```python
from build123d import *

# Parameters (mm, degrees)
SKETCH1_R           = 22.4995417
SKETCH1_R_2         = 17.4995417
BOSS_EXTRUDE1_DEPTH = 6
CUT_EXTRUDE1_START  = -4
SKETCH2_R           = 19.4995417
SKETCH2_R_2         = 17.4995417
CUT_EXTRUDE1_DEPTH  = 4
BOSS_EXTRUDE2_DEPTH = 6
BOSS_EXTRUDE3_START = 24
BOSS_EXTRUDE3_DEPTH = 24
BOSS_EXTRUDE4_START = 5
SKETCH6_R           = 22.4995417
SKETCH6_R_2         = 8.79453705
BOSS_EXTRUDE4_DEPTH = 5
CUT_EXTRUDE2_DEPTH  = 50
SKETCH8_W           = 26.34206851
SKETCH8_H           = 62.78523096
CUT_EXTRUDE3_DEPTH  = 44.051814752
SKETCH9_R           = 2.165
CUT_EXTRUDE4_DEPTH  = 33.379912807


with BuildPart() as part:
    # Sketch1 → Boss-Extrude1 (new body)
    with BuildSketch(Plane.XY):
        Circle(SKETCH1_R)
        Circle(SKETCH1_R_2, mode=Mode.SUBTRACT)
    extrude(amount=BOSS_EXTRUDE1_DEPTH)

    # Sketch2 → Cut-Extrude1 (cut)
    with BuildSketch(Plane.XY.offset(6).offset(CUT_EXTRUDE1_START)):
        Circle(SKETCH2_R)
        Circle(SKETCH2_R_2, mode=Mode.SUBTRACT)
    extrude(amount=CUT_EXTRUDE1_DEPTH, mode=Mode.SUBTRACT)

    # Sketch3 → Boss-Extrude2 (add, through all)
    with BuildSketch(Plane(origin=(0, 0, 0), x_dir=(-1, 0, 0), z_dir=(0, 0, -1))):
        with BuildLine():
            Line((-7.783576547, 21.11031295), (-21.864631522, 21.11031295))
            Line((-21.864631522, 21.11031295), (-21.864631522, 5.307284156))
            ThreePointArc((-21.864631522, 5.307284156), (-16.798452018, 14.96801211), (-7.783576547, 21.11031295))
        make_face()
        with BuildLine():
            Line((21.864631522, -21.11031295), (7.783576547, -21.11031295))
            ThreePointArc((7.783576547, -21.11031295), (16.798452018, -14.96801211), (21.864631522, -5.307284156))
            Line((21.864631522, -5.307284156), (21.864631522, -21.11031295))
        make_face()
        with BuildLine():
            Line((21.864631522, 21.11031295), (7.783576547, 21.11031295))
            ThreePointArc((7.783576547, 21.11031295), (16.798452018, 14.96801211), (21.864631522, 5.307284156))
            Line((21.864631522, 5.307284156), (21.864631522, 21.11031295))
        make_face()
        with BuildLine():
            Line((-21.864631522, -21.11031295), (-21.864631522, -5.307284156))
            ThreePointArc((-21.864631522, -5.307284156), (-16.798452018, -14.96801211), (-7.783576547, -21.11031295))
            Line((-7.783576547, -21.11031295), (-21.864631522, -21.11031295))
        make_face()
    extrude(amount=-BOSS_EXTRUDE2_DEPTH)

    # Sketch5 → Boss-Extrude3 (add)
    with BuildSketch(Plane(origin=(0, 0, 0), x_dir=(-1, 0, 0), z_dir=(0, 0, -1)).offset(BOSS_EXTRUDE3_START)):
        with BuildLine():
            Line((-14.441527519, 9.883129191), (-18.5677863, 12.706954341))
            ThreePointArc((-18.5677863, 12.706954341), (-22.4995417, 0), (-18.5677863, -12.706954341))
            Line((-18.5677863, -12.706954341), (-14.441527519, -9.883129191))
            ThreePointArc((-14.441527519, -9.883129191), (-17.4995417, 0), (-14.441527519, 9.883129191))
        make_face()
    extrude(amount=-BOSS_EXTRUDE3_DEPTH)

    # Sketch6 → Boss-Extrude4 (add)
    with BuildSketch(Plane(origin=(0, 0, -24), x_dir=(-1, 0, 0), z_dir=(0, 0, -1)).offset(BOSS_EXTRUDE4_START)):
        Circle(SKETCH6_R)
        Circle(SKETCH6_R_2, mode=Mode.SUBTRACT)
    extrude(amount=-BOSS_EXTRUDE4_DEPTH)

    # Sketch7 → Cut-Extrude2 (cut, symmetric)
    with BuildSketch(Plane(origin=(0, 0, 0), x_dir=(-1, 0, 0), z_dir=(0, 0, -1))):
        Polygon((0, 20.425006128), (0, -31.813494394), (-34.413040629, -24.963896379), (-30.369302041, 32.308646058), (-0.660202218, 29.585311907), (0, 25.789149152), align=None)
    extrude(amount=CUT_EXTRUDE2_DEPTH, both=True, mode=Mode.SUBTRACT)


with BuildPart() as cut_extrude2_piece_1:
    # of the separate pieces the step leaves, piece 1, a body of its own (cut_extrude2_pieces)
    add(part.part.solids().sort_by_distance((0, -22.4995417, -24))[0])

    # Sketch8 → Cut-Extrude3 (cut, through all)
    with BuildSketch(Plane(origin=(0, 0, 0), x_dir=(0, 0, -1), z_dir=(1, 0, 0))):
        with Locations((23.482670262, -0.940788161)):
            Rectangle(SKETCH8_W, SKETCH8_H)
    extrude(amount=-CUT_EXTRUDE3_DEPTH, mode=Mode.SUBTRACT)


with BuildPart() as cut_extrude2_piece_2:
    # of the separate pieces the step leaves, piece 2, a body of its own (cut_extrude2_pieces)
    add(part.part.solids().sort_by_distance((0, 17.4995417, 0))[0])

    # Sketch9 → Cut-Extrude4 (cut, through all)
    with BuildSketch(Plane(origin=(0, 0, 0), x_dir=(-1, 0, 0), z_dir=(0, 0, -1))):
        with Locations((16.571715691, 16)):
            Circle(SKETCH9_R)
        with Locations((16.571715691, -16)):
            Circle(SKETCH9_R)
        with Locations((-16.571715691, -16)):
            Circle(SKETCH9_R)
        with Locations((-16.571715691, 16)):
            Circle(SKETCH9_R)
    extrude(amount=-CUT_EXTRUDE4_DEPTH, mode=Mode.SUBTRACT)


solid = cut_extrude2_piece_2.part
```
Check sheet for the modelled part. Datum: model origin and axes. Units: mm. A direction names the side the tool comes from. Round coordinates to 2 decimals unless told otherwise and drop trailing zeros. Order: outer loops, then holes, each group sorted by start corner. A loop starts at its lowest first (then second) coordinate and runs counter-clockwise, first axis right, second up. Notation, with made-up numbers: M 22,58.5 L 61,58.5 A14 ccw 61,66.5 Z; hole C -39.75,47 d7. An arc over 180 degrees is marked long. Answer in a Markdown table with one row per item.
(1) Gauge pin test, flat ends, axial feed: pin 1 (2 mm diameter, centred on x = -11.5, z = 2, fed in from -Y); pin 2 (1.8 mm diameter, centred on y = -9.5, z = 3, fed in from -X); pin 3 (2 mm diameter, centred on y = 3, z = 1.5, fed in from -X); pin 4 (3.5 mm diameter, centred on x = -16.57, y = 16, fed in from -Z). Record the tip position at first contact, or that the pin passes through.
Findings:
| item | result |
|---|---|
| pin 1 | stops at y = -21.11 |
| pin 2 | stops at x = -21.86 |
| pin 3 | stops at x = -22.41 |
| pin 4 | passes through |
(2) Section check D-D on y = 0. Record the boundary of the cut face in (x, z), plus the area to 3 significant figures.
Findings:
| item | result |
|---|---|
| outline | M -22.5,0 L -17.5,0 L -17.5,2 L -19.5,2 L -19.5,6 L -22.5,6 Z |
| area | 22.0 mm^2 |
(3) Material ranges on line 1 along Y through (x, z) = (-15, 3.75); line 2 along Y through (x, z) = (-16, 2.2); line 3 along Y through (x, z) = (-20.75, 4.25), recorded low to high. Write a range as from..to.
Findings:
| item | result |
|---|---|
| line 1 | y = -21.11..-17.49, -14.51..-12.46, 12.46..14.51, 17.49..21.11 |
| line 2 | y = -21.11..-18.09, -13.91..-11.15, 11.15..13.91, 18.09..21.11 |
| line 3 | y = -21.11..21.11 |
(4) Draft check along Y on faces 1 (the cylindrical face through (-17.495, 0.385, 0.986)), 2 (the flat face through (-15, 21.11, 3)), 3 (the flat face through (-15, -21.11, 3)), 4 (the flat face through (-19, 0, 0)). Enter one of: +Y half, -Y half, draft (parallel to the pull), parting line (faces both ways), or undercut.
Findings:
| item | result |
|---|---|
| face 1 | undercut |
| face 2 | +Y half |
| face 3 | -Y half |
| face 4 | draft |
(5) Set-up check for faces 5 (the flat face through (-21.865, 13, 3)), 6 (the flat face through (-21.865, -13, 3)), 7 (the cylindrical face through (-22.5, 0.1, 3)), 8 (the cylindrical face through (-19.495, 0.429, 3.972)): record each of +Z, -Z, +X, -X, +Y, -Y from which the full face is reachable in a straight line by a thin tool's end or side.
Findings:
| item | result |
|---|---|
| face 5 | +Z, -Z, -X, +Y |
| face 6 | +Z, -Z, -X, -Y |
| face 7 | +Z, -Z, -X |
| face 8 | +Z, +X |
(6) Section check B-B on z = 5.5. Record the boundary of the cut face in (x, y) (3 decimals).
Findings:
| item | result |
|---|---|
| outline | M -21.865,-21.11 L -7.784,-21.11 A22.5 ccw 0,-22.5 L 0,-19.5 A19.5 cw 0,19.5 L 0,22.5 A22.5 ccw -7.784,21.11 L -21.865,21.11 L -21.865,5.307 A22.5 ccw -21.865,-5.307 Z; hole C -16.572,-16 d4.33; hole C -16.572,16 d4.33 |
(7) Section check C-C on y = -16. Record the boundary of the cut face in (x, z).
Findings:
| item | result |
|---|---|
| outline | M -21.86,0 L -18.74,0 L -18.74,6 L -21.86,6 Z; M -14.41,0 L -7.09,0 L -7.09,2 L -11.15,2 L -11.15,6 L -14.41,6 Z |
(8) Section check A-A on x = -2.5. Record the boundary of the cut face in (y, z), plus the area to 3 significant figures.
Findings:
| item | result |
|---|---|
| outline | M -22.36,0 L -17.32,0 L -17.32,2 L -19.34,2 L -19.34,6 L -22.36,6 Z; M 17.32,0 L 22.36,0 L 22.36,6 L 19.34,6 L 19.34,2 L 17.32,2 Z |
| area | 44.3 mm^2 |
